Verification items for the finished model (mm, model axes). Face numbers are marked on the shaded views. A direction names the side the tool comes from. Round coordinates to 2 decimals unless told otherwise and drop trailing zeros. Write each loop counter-clockwise with the first axis right and the second up, starting at its lowest first coordinate (ties: lowest second). Pieces come first, ordered by that corner, then holes. Notation, with made-up numbers: M 33,-8 L 62,-8 A14 cw 62,3 Z; hole C -6.75,-21 d5. An arc over 180 degrees is marked long. One line per question, with ' | ' between items. Start each with the question number.
Q1. Thickness scan on line 1 along Y through (x, z) = (-20.5, -0.75); line 2 along Y through (x, z) = (-24, 0); line 3 along Y through (x, z) = (-13, 5.25). Record the ranges inside material, lowest first. Write a range as from..to.
Q2. Cross-section at A-A (y = 8). Record the boundary of the cut face in (x, z), then the cut area to 3 significant figures.
Q3. Release check for a two-part mould opening along Y. For the marked faces 1, 2 and 3 record: released by +Y, released by -Y, zero draft, split by the parting line, or undercut.
Q4. Tool access check on the marked faces 4 and 5. Record the directions out of +Z, -Z, +X, -X, +Y, -Y that give a thin tool (end or side, any length) a straight path to the whole face; none if there is none.
Q5. Cross-section at B-B (z = -1.5). Record the boundary of the cut face in (x, y), then the cut area to 3 significant figures.
Q6. Cross-section at D-D (z = 3.75). Record the boundary of the cut face in (x, y).
Q7. Gauge pin test, flat ends, axial feed: pin 1 (3 mm diameter, centred on x = -23.5, z = -2.5, fed in from +Y); pin 2 (6 mm diameter, centred on x = -5.5, z = -2, fed in from -Y); pin 3 (2 mm diameter, centred on x = -25, y = 17, fed in from -Z). Record the tip position at first contact, or that the pin passes through.
Q8. Cross-section at C-C (x = -14.5). Record the boundary of the cut face in (y, z), then the cut area to 3 significant figures.
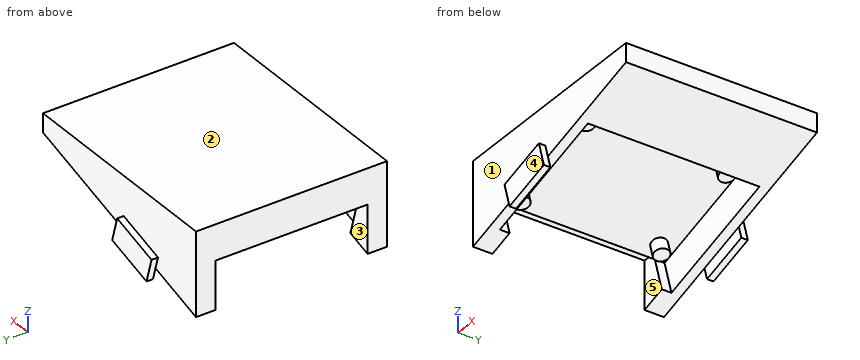
from build123d import *

# Parameters (mm, degrees)
BOSS_EXTRUDE1_DEPTH = 29.5
SKETCH2_W           = 20.5
SKETCH2_H           = 26.5
CUT_EXTRUDE1_DEPTH  = 5.5
CUT_EXTRUDE2_REACH  = 36.22
SKETCH3_W           = 7.420012267
SKETCH3_H           = 23.5
SKETCH4_R           = 1.15
BOSS_EXTRUDE2_DEPTH = 2
BOSS_EXTRUDE3_DEPTH = 1
BOSS_EXTRUDE4_DEPTH = 1


with BuildPart() as part:
    # Sketch1 → Boss-Extrude1 (new body)
    with BuildSketch(Plane(origin=(0, 0, 0), x_dir=(1, 0, 0), z_dir=(0, 1, 0))):
        Polygon((-25.843422974, -5.060047824), (-25.843422974, 4.909964443), (8.376577026, -5.060047824), (8.376577026, -7.960047824), (-25.843422974, -7.960047824), align=None)
    extrude(amount=BOSS_EXTRUDE1_DEPTH)

    # Sketch2 → Cut-Extrude1 (cut)
    with BuildSketch(Plane(origin=(-0.703485348, 0, 2.414567601), x_dir=(-0.960081566, 0, -0.279720193), z_dir=(0.279720193, 0, -0.960081566))):
        with Locations((11.935210206, 14.75)):
            Rectangle(SKETCH2_W, SKETCH2_H)
    extrude(amount=-CUT_EXTRUDE1_DEPTH, mode=Mode.SUBTRACT)

    # Cut-Extrude2: up to this face of the body (flat: up to its plane)
    cut_extrude2_end = Plane(part.part.faces().sort_by_distance((-22.772327239, 14.75, -1.150859365))[0])
    # Sketch3 → Cut-Extrude2 (cut, up to the picked face)
    with BuildSketch(Plane.ZY.offset(25.843422974), mode=Mode.PRIVATE) as cut_extrude2_sk1:
        with Locations((-1.19995831, 14.75)):
            Rectangle(SKETCH3_W, SKETCH3_H)
    cut_extrude2_tool1 = split(extrude(cut_extrude2_sk1.sketch, amount=-CUT_EXTRUDE2_REACH, mode=Mode.PRIVATE), bisect_by=cut_extrude2_end, keep=Keep.BOTH, mode=Mode.PRIVATE)
    add(cut_extrude2_tool1.solids().sort_by_distance((-25.843423, 14.75, -1.199958))[0], mode=Mode.SUBTRACT)

    # Sketch4 → Boss-Extrude2 (add)
    with BuildSketch(Plane(origin=(-2.241946407, 0, 7.695016215), x_dir=(-0.960081566, 0, -0.279720193), z_dir=(0.279720193, 0, -0.960081566))):
        with Locations((19.685210206, 25.5)):
            Circle(SKETCH4_R)
        with Locations((19.685210206, 3.9)):
            Circle(SKETCH4_R)
        with Locations((4.485210206, 3.9)):
            Circle(SKETCH4_R)
        with Locations((4.485210206, 25.5)):
            Circle(SKETCH4_R)
    extrude(amount=BOSS_EXTRUDE2_DEPTH)

    # Sketch5 → Boss-Extrude3 (add)
    with BuildSketch(Plane(origin=(0, 0, 0), x_dir=(-1, 0, 0), z_dir=(0, -1, 0))):
        Polygon((9.662770444, -1.887432229), (17.343422974, 0.350329313), (16.224542204, 4.190655577), (8.543889674, 1.952894036), align=None)
    extrude(amount=BOSS_EXTRUDE3_DEPTH)

    # Sketch6 → Boss-Extrude4 (add)
    with BuildSketch(Plane(origin=(0, 29.5, 0), x_dir=(1, 0, 0), z_dir=(0, 1, 0))):
        Polygon((-16.224542204, 4.190655577), (-8.543889674, 1.952894036), (-9.662770444, -1.887432229), (-17.343422974, 0.350329313), align=None)
    extrude(amount=BOSS_EXTRUDE4_DEPTH)


solid = part.part
Determined:
1) line 1: y = 0..1.5, 28..29.5 | line 2: y = 0..3, 26.5..29.5 | line 3: y = 0..29.5
2) outline: M -25.84,2.51 L -23.84,2.51 L -23.54,1.49 L -3.86,7.22 L -2.32,1.94 L 8.38,5.06 L 8.38,7.96 L -25.84,7.96 Z | area: 137 mm²
3) face 1: released by -Y | face 2: zero draft | face 3: undercut
4) face 4: +Z, -Z, +X, -X, -Y | face 5: -Z, -X
5) outline: M -25.84,0 L -17.01,0 L -17.01,-1 L -8.68,-1 L -8.68,0 L -14.14,0 L -14.14,1.5 L -22.67,1.5 L -22.67,3 L -25.84,3 Z; M -25.84,26.5 L -22.67,26.5 L -22.67,28 L -14.14,28 L -14.14,29.5 L -8.68,29.5 L -8.68,30.5 L -17.01,30.5 L -17.01,29.5 L -25.84,29.5 Z | area: 61.3 mm²
6) outline: M -25.84,0 L 3.88,0 L 3.88,29.5 L -25.84,29.5 Z; hole M -15.78,1.5 L -2.85,1.5 L -2.85,28 L -15.78,28 Z
7) pin 1: stops at y = 29.5 | pin 2: stops at y = 0 | pin 3: stops at z = 2.51
8) outline: M -1,-3.69 L 0,-3.69 L 0,-1.61 L 1.5,-1.61 L 1.5,4.12 L 28,4.12 L 28,-1.61 L 29.5,-1.61 L 29.5,-3.69 L 30.5,-3.69 L 30.5,0.48 L 29.5,0.48 L 29.5,7.96 L 0,7.96 L 0,0.48 L -1,0.48 Z | area: 139 mm²
